CAD build for the part. Positions are in the model's coordinates, mm. Face numbers are marked on the shaded views. A direction names the side the tool comes from. Give positions to 0.01 mm unless a question says otherwise; leave off trailing zeros. Use one line per item in the form item = value. Start each with the question number.
from build123d import *

# Parameters (mm, degrees)
F0_R     = 39.683512
F1_DEPTH = 21.09801
F2_R     = 20.955301
F3_R     = 4.810594
F4_DEPTH = 3.81
F5_R     = 4.782773
F6_DEPTH = 6.43239


with BuildPart() as f1:
    # F0 (on Front) → F1 (new body)
    with BuildSketch(Plane.XZ):
        Circle(F0_R)
    extrude(amount=-F1_DEPTH)

    # F2
    f2_edges = [f1.edges().sort_by_distance(p)[0] for p in [
        (-39.683512, 21.09801, 0),
    ]]
    fillet(f2_edges, radius=F2_R)

    # F3 (on Right) → F4 (join, symmetric)
    with BuildSketch(Plane.YZ):
        with BuildLine():
            ThreePointArc((14.871401, -19.424973), (28.639419, -13.722073), (34.342318, 0.045945))
            ThreePointArc((34.342318, 0.045945), (28.639419, 13.813962), (14.871401, 19.516862))
            Line((14.871401, 19.516862), (14.871401, 0.045945))
            Line((14.871401, 0.045945), (14.871401, -19.424973))
        make_face()
        with Locations((27.04107, 0)):
            Circle(F3_R, mode=Mode.SUBTRACT)
    extrude(amount=F4_DEPTH, both=True)

    # F5 (on Right) → F6 (join, symmetric)
    with BuildSketch(Plane.YZ):
        with Locations((26.935229, 0)):
            Circle(F5_R)
    extrude(amount=F6_DEPTH, both=True)


solid = f1.part
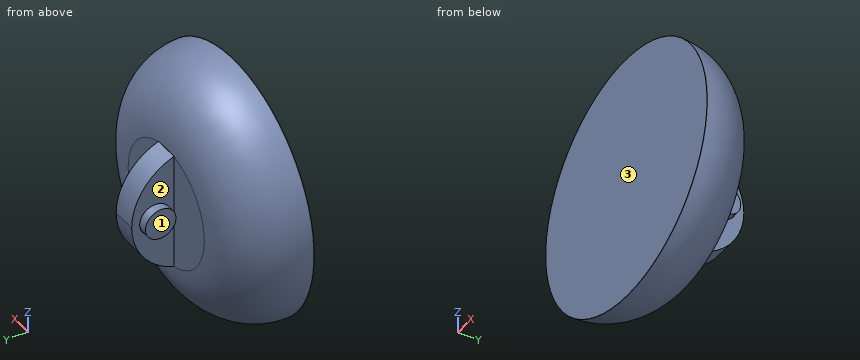
1) Wall check: line 1 along X through (y, z) = (32.5, -4); line 2 along Y through (x, z) = (11.5, 10); line 3 along Y through (x, z) = (-23, -18.5). Give the ranges that are in metal, low to high. Write a range as from..to.
2) 3-axis set-ups, long thin cutter, end or side, ignore diameter. For the marked faces 1, 2 and 3: which of +Z, -Z, +X, -X, +Y, -Y reach the whole face in a straight line?
3) Pin check, flat tips, straight feed: pin 1 (6 mm diameter, centred on y = 26.5, z = 15.5, fed in from -X); pin 2 (10.5 mm diameter, centred on y = 30, z = -1, fed in from -X); pin 3 (5 mm diameter, centred on y = 5, z = -5.5, fed in from -X); pin 4 (16.5 mm diameter, centred on x = 8.5, z = -2.5, fed in from +Y). Stop position of each tip, or through.
Final values:
q1.line_1 = -3.81..3.81
q1.line_2 = 0..21.1
q1.line_3 = 0..18.11
q2.face_1 = +Z, -Z, -X, +Y
q2.face_2 = -X
q2.face_3 = +Z, -Z, +X, -X, -Y
q3.pin_1 = -3.81
q3.pin_2 = -6.43
q3.pin_3 = -39.28
q3.pin_4 = 34.34
